The listing builds one solid part. Answer for the finished solid, in the listing's coordinates (mm). A direction names the side the tool comes from. Give positions to 0.01 mm unless a question says otherwise; leave off trailing zeros. Loops run counter-clockwise (first coordinate to the right, second up) from the corner with the lowest first, then second, coordinate; pieces in that order, holes last. Notation, with made-up numbers: (72.5, -16.5) - (122.5, -16.5) arc R33 cw to (122.5, 20.5) - close; hole circle Ø6 at (13, 55). An arc over 180 degrees is marked (long way). Write each question's results on one line, items separated by ' | '.
Autodesk Inventor part; units mm, degrees
ref_plane "YZ Plane" through (0, 0, 0) normal (1, 0, 0) x (0, 1, 0)
ref_plane "XZ Plane" through (0, 0, 0) normal (0, 1, 0) x (-1, 0, 0)
ref_plane "XY Plane" through (0, 0, 0) normal (0, 0, 1) x (1, 0, 0)
sketch "Sketch1" plane through (0, 0, 0) normal (0, 0, 1) x (1, 0, 0)
  line L0 (50.5181, -87.5) -> (-50.5181, -87.5)
  line L1 (-50.5181, -87.5) -> (-101.0363, 0)
  line L2 (-101.0363, 0) -> (-50.5181, 87.5)
  line L3 (-50.5181, 87.5) -> (50.5181, 87.5)
  line L4 (50.5181, 87.5) -> (101.0363, 0)
  line L5 (101.0363, 0) -> (50.5181, -87.5)
  point P0 (0, 0)
  point P1 (0, 0)
  dimension "d0" = 175
extrude "Extrusion1" add sketch "Sketch1" along normal blind 2
sketch "Sketch7" plane through (0, 0, 2) normal (0, 0, 1) x (1, 0, 0)
  line L0 (-50.5181, -87.5) -> (50.5181, -87.5)
  line L1 (50.5181, -87.5) -> (101.0363, 0)
  line L2 (101.0363, 0) -> (50.5181, 87.5)
  line L3 (50.5181, 87.5) -> (-50.5181, 87.5)
  line L4 (-50.5181, 87.5) -> (-101.0363, 0)
  line L5 (-101.0363, 0) -> (-50.5181, -87.5)
  line L6 (-47.054, 81.5) -> (47.054, 81.5)
  line L7 (47.054, 81.5) -> (94.1081, 0)
  line L8 (94.1081, 0) -> (47.054, -81.5)
  line L9 (47.054, -81.5) -> (-47.054, -81.5)
  line L10 (-47.054, -81.5) -> (-94.1081, 0)
  line L11 (-94.1081, 0) -> (-47.054, 81.5)
  dimension "d26" = 6
extrude "Extrusion6" cut sketch "Sketch7" against normal blind 7 contours L6 L7 L8 L9 L10 L11
fillet "Fillet2" radius 10 6 edges at (-94.1081, 0, 1) (-47.054, -81.5, 1) (47.054, -81.5, 1) (94.1081, 0, 1) (47.054, 81.5, 1) (-47.054, 81.5, 1)
fillet "Fillet3" radius 10 6 edges at (-50.5181, 87.5, 1) (50.5181, 87.5, 1) (101.0363, 0, 1) (50.5181, -87.5, 1) (-50.5181, -87.5, 1) (-101.0363, 0, 1)
properties part number "Cover v1"
Item 1: Find the intervals of material crossed by line 1 along Y through (x, z) = (18, 0.45); line 2 along X through (y, z) = (-38, 0.8); line 3 along X through (y, z) = (-3, 1.05), in increasing order. Write a range as [from, to].
Values found:
line 1: y = [-87.5, -81.5], [81.5, 87.5] | line 2: x = [-79.1, -72.17], [72.17, 79.1] | line 3: x = [-99.03, -92.1], [92.1, 99.03]
Item 2: A cutting plane is placed at C-C, the plane y = 32. Determine the outline of the cut face in (x, z), plus the area to 3 significant figures.
Values found:
outline: (-82.56, 0) - (-75.63, 0) - (-75.63, 2) - (-82.56, 2) - close; (75.63, 0) - (82.56, 0) - (82.56, 2) - (75.63, 2) - close | area: 27.7 mm²
Item 3: A flat-ended cylindrical pin translates along its axis: P1, Ø1, axis at y = -23, z = 1, coming from the -X side. Find the tip coordinate at first contact, or state that the pin passes through.
Values found:
P1: stops at x = -88.05
Item 4: A cutting plane is placed at B-B, the plane x = 31.5. Determine the outline of the cut face in (y, z).
Values found:
outline: (-87.5, 0) - (-81.5, 0) - (-81.5, 2) - (-87.5, 2) - close; (81.5, 0) - (87.5, 0) - (87.5, 2) - (81.5, 2) - close
Item 5: For faces 1 (the face through (-49.681, 86.197, 1.014)), 2 (the face through (46.344, -80.123, 0.986)), determine the directions among +Z, -Z, +X, -X, +Y, -Y from which every point of the face is accessible in a straight line to the end or side of a thin tool.
Values found:
face 1: +Z, -Z, -X, +Y | face 2: +Z, -Z
Item 6: A cutting plane is placed at A-A, the plane z = 1.3. Determine the outline of the cut face in (x, y).
Values found:
outline: (-98.15, -5) - (-53.4, -82.5) arc R10 ccw to (-44.74, -87.5) - (44.74, -87.5) arc R10 ccw to (53.4, -82.5) - (98.15, -5) arc R10 ccw to (98.15, 5) - (53.4, 82.5) arc R10 ccw to (44.74, 87.5) - (-44.74, 87.5) arc R10 ccw to (-53.4, 82.5) - (-98.15, 5) arc R10 ccw to start; hole (-91.22, -5) - (-49.94, -76.5) arc R10 ccw to (-41.28, -81.5) - (41.28, -81.5) arc R10 ccw to (49.94, -76.5) - (91.22, -5) arc R10 ccw to (91.22, 5) - (49.94, 76.5) arc R10 ccw to (41.28, 81.5) - (-41.28, 81.5) arc R10 ccw to (-49.94, 76.5) - (-91.22, 5) arc R10 ccw to start
Item 7: For a pull along Y with two mould halves and no side action, classify faces 3 (the face through (49.681, -86.197, 1.014)), 4 (the face through (46.217, 80.197, 0.986)), 5 (the face through (70.9, -40.2, 1)), 6 (the face through (-76.09, 43.21, 0.99)) as released by +Y, released by -Y, zero draft, split by the parting line, or undercut.
Values found:
face 3: released by -Y | face 4: undercut | face 5: undercut | face 6: released by +Y
